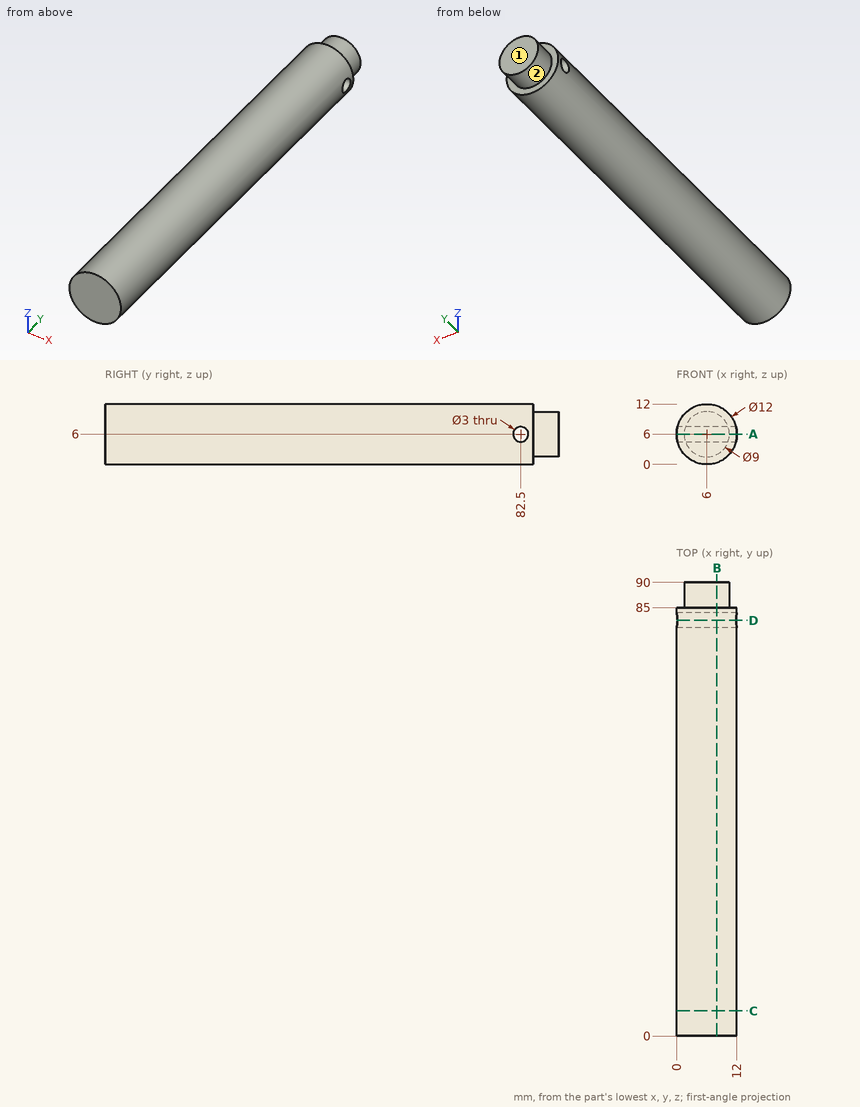
Source: three-view drawing plus pictorial views. Frame: mm from the lowest corner of the part. A direction names the side the tool comes from. Round coordinates to 2 decimals unless told otherwise and drop trailing zeros. Loops run counter-clockwise (first coordinate to the right, second up) from the corner with the lowest first, then second, coordinate; pieces in that order, holes last.
1. Section query B-B on x = 8. Output: boundary loops of the cut face in (y, z), and give its area (3 significant figures).
2. Section query C-C on y = 5. Output: boundary loops of the cut face in (x, z).
3. Contact query for flat-ended pins moving along their axis: pin 1 (5 mm diameter, centred on y = 59, z = 9, fed in from -X); pin 2 (3 mm diameter, centred on x = 10, y = 54.5, fed in from +Z); pin 3 (6 mm diameter, centred on x = 2.5, y = 20.5, fed in from -Z). Output: stop coordinate, or through.
4. Section query A-A on z = 6. Output: boundary loops of the cut face in (x, y).
5. Ray query, L1, parallel to Y at x = 9, z = 6; L2, parallel to Y at x = 6.75, z = 11.5; L3, parallel to Z at x = 9.75, y = 83.5. Return the intervals inside material, ascending.
6. Section query D-D on y = 82.5. Output: boundary loops of the cut face in (x, z), and give its area (3 significant figures).
7. Access query for the marked faces 1 and 2. Directions: +Z, -Z, +X, -X, +Y, -Y. A direction counts if a zero-diameter tool reaches every point of the face in a straight line with its end or side. Return the directions, or none.
Answers below:
1. outline: (0, 0.34) - (85, 0.34) - (85, 1.97) - (90, 1.97) - (90, 10.03) - (85, 10.03) - (85, 11.66) - (0, 11.66) - close; hole circle Ø3 at (82.5, 6)
1. area: 995 mm2
2. outline: circle Ø12 at (6, 6)
3. pin 1: stops at x = 0.02
3. pin 2: stops at z = 11.45
3. pin 3: stops at z = 0.02
4. outline: (0, 0) - (12, 0) - (12, 81) - (0, 81) - close; (0, 84) - (12, 84) - (12, 85) - (10.5, 85) - (10.5, 90) - (1.5, 90) - (1.5, 85) - (0, 85) - close
5. L1: y = 0 to 81, 84 to 90
5. L2: y = 0 to 85
5. L3: z = 1.32 to 4.88, 7.12 to 10.68
6. outline: (0.19, 4.5) arc R6 ccw to (11.81, 4.5) - close; (0.19, 7.5) - (11.81, 7.5) arc R6 ccw to start
6. area: 77.5 mm2
7. face 1: +Z, -Z, +X, -X, +Y
7. face 2: +Y
